Can you work these out from the model? Positions are in its coordinate system, mm. A direction names the side the tool comes from. Round coordinates to 2 decimals unless told otherwise and drop trailing zeros. Loops run counter-clockwise (first coordinate to the right, second up) from the corner with the lowest first, then second, coordinate; pieces in that order, holes last.
from build123d import *

# Parameters (mm, degrees)
BOSS_EXTRUDE1_DEPTH  = 3.175
SKETCH3_W            = 3.2258
SKETCH3_H            = 6.35
HOLES_FOR_TABS_DEPTH = 4.1750001


with BuildPart() as part:
    # Sketch1 → Boss-Extrude1 (new body)
    with BuildSketch(Plane.XY):
        with BuildLine():
            Line((-76.2, 43.18), (-37.713355451, 36.56692496))
            Line((-37.713355451, 36.56692496), (0, 35.56))
            Line((0, 35.56), (0, 0))
            Line((0, 0), (-143.94013079, 0))
            Line((-143.94013079, 0), (-137.895807931, 35.176631753))
            Line((-137.895807931, 35.176631753), (-129.892439684, 43.18))
            add(Edge.make_bspline(
                [(-129.892439684, 43.18), (-123.632909294, 45.955986916), (-114.625709488, 48.362317243), (-103.247996656, 48.972136691), (-95.522501134, 48.59342086), (-86.411542659, 47.027463229), (-79.726058772, 44.740816459), (-76.2, 43.18)],
                knots=[0, 0, 0, 0, 0.371232541, 0.49990694, 0.617608528, 0.790714497, 1, 1, 1, 1], degree=3))
        make_face()
    extrude(amount=BOSS_EXTRUDE1_DEPTH)

    # Sketch3 → holes for tabs (cut, through all)
    with BuildSketch(Plane.XY.offset(3.175)):
        with Locations((-36.6649, 27.305)):
            Rectangle(SKETCH3_W, SKETCH3_H)
        with Locations((-36.6649, 8.255)):
            Rectangle(SKETCH3_W, SKETCH3_H)
    extrude(amount=-HOLES_FOR_TABS_DEPTH, mode=Mode.SUBTRACT)


solid = part.part
(1) If we section it at C-C, the plane y = 6.5: List the corners of the cut face in (x, z) for me (3 decimals).
Worked answers:
outline: (-142.823, 0) - (-38.278, 0) - (-38.278, 3.175) - (-142.823, 3.175) - close; (-35.052, 0) - (0, 0) - (0, 3.175) - (-35.052, 3.175) - close
(2) If we mould it in two halves opening along Y, with no side actions, what happens to faces 3 (the flat face through (-71, 0, 2)), 4 (the flat face through (-37, 5.08, 2)), 5 (the flat face through (0, 18, 2)), 6 (the flat face through (-57.23, 39.92, 1.57))? For each: released by +Y, released by -Y, zero draft, split by the parting line, or undercut.
Worked answers:
face 3: released by -Y
face 4: undercut
face 5: zero draft
face 6: released by +Y
(3) For faces 1 (the flat face through (-37, 24.13, 2)), 2 (the flat face through (-140.96, 17.34, 1.57)), which set-ups out of +Z, -Z, +X, -X, +Y, -Y let a thin tool reach every point of the face, with its end or its side?
Worked answers:
face 1: +Z, -Z
face 2: +Z, -Z, -X, +Y
(4) Will these pins go through, and if not, where does the flat tip stop? P1, Ø1, axis at y = 29, z = 2.5, coming from the -X side; P2, Ø4, axis at x = -104, y = 20.5, coming from the -Z side; P3, Ø1.6, axis at x = -36.5, z = 1, coming from the +Y side.
Worked answers:
P1: stops at x = -139.04
P2: stops at z = 0
P3: stops at y = 36.56
(5) If we section it at A-A, the plane y = 29: List the corners of the cut face in (x, z) for me (3 decimals).
Worked answers:
outline: (-138.957, 0) - (-38.278, 0) - (-38.278, 3.175) - (-138.957, 3.175) - close; (-35.052, 0) - (0, 0) - (0, 3.175) - (-35.052, 3.175) - close
(6) If we section it at B-B, the plane z = 1.65: State how many separate pieces and enclosed holes the cut face has, then the cut area to 3 significant figures.
Worked answers:
separate pieces: 1
enclosed holes: 2
area: 5,800 mm2
(7) If I drill on line 1 (X direction, y = 10, z = 1.3); line 2 (X direction, y = 35, z = 3.05); line 3 (X direction, y = 34, z = 1), over which ranges is the centre line in solid material (lowest first)?
Worked answers:
line 1: x = -142.22 to -38.28, -35.05 to 0
line 2: x = -137.93 to 0
line 3: x = -138.1 to 0
(8) If we section it at D-D, the plane x = -9: List the corners of the cut face in (y, z) for me (3 decimals).
Worked answers:
outline: (0, 0) - (35.8, 0) - (35.8, 3.175) - (0, 3.175) - close
